from build123d import *

# Parameters (mm, degrees)
F0_R      = 20
F1_DEPTH  = 5
F2_R      = 16.6
F3_DEPTH  = 5
F4_W      = 6
F4_H      = 11
F5_DEPTH  = 2.5
F6_R      = 2
F7_SIZE   = 3
F8_W      = 2.95381
F8_H      = 3.5
F9_DEPTH  = 2.5
F10_R     = 1.25
F12_DEPTH = 0.75
F13_R     = 0.545211
F15_R     = 17.3
F15_R_2   = 16.6
F16_DEPTH = 5


with BuildPart() as f1:
    # F0 (on Top) → F1 (new body)
    with BuildSketch(Plane.XY):
        Circle(F0_R)
    extrude(amount=F1_DEPTH)

    # F2 (on face) → F3 (join)
    with BuildSketch(Plane.XY.offset(5)):
        Circle(F2_R)
    extrude(amount=F3_DEPTH)

    # F4 (on face) → F5 (join)
    with BuildSketch(Plane(origin=(0, 0, 0), x_dir=(1, 0, 0), z_dir=(0, 0, -1))):
        with Locations((0, -7.136372)):
            Rectangle(F4_W, F4_H)
    extrude(amount=F5_DEPTH)

    # F6
    f6_edges = [f1.edges().sort_by_distance(p)[0] for p in [
        (-3, 12.636372, -1.25),
        (3, 12.636372, -1.25),
        (3, 1.636372, -1.25),
        (-3, 1.636372, -1.25),
    ]]
    fillet(f6_edges, radius=F6_R)

    # F7
    f7_edges = [f1.edges().sort_by_distance(p)[0] for p in [
        (-20, 0, 0),
    ]]
    chamfer(f7_edges, length=F7_SIZE)

    # F8 (on face) → F9 (cut)
    with BuildSketch(Plane(origin=(0, 0, -2.5), x_dir=(1, 0, 0), z_dir=(0, 0, -1))):
        with Locations((0, -4.806658)):
            Rectangle(F8_W, F8_H)
        with Locations((0, -9.536388)):
            Rectangle(F8_W, F8_H)
    extrude(amount=-F9_DEPTH, mode=Mode.SUBTRACT)

    # F10
    f10_edges = [f1.edges().sort_by_distance(p)[0] for p in [
        (1.476905, 3.056658, -1.25),
        (-1.476905, 3.056658, -1.25),
        (1.476905, 6.556658, -1.25),
        (-1.476905, 6.556658, -1.25),
        (1.476905, 7.786388, -1.25),
        (-1.476905, 7.786388, -1.25),
        (-1.476905, 11.286388, -1.25),
        (1.476905, 11.286388, -1.25),
    ]]
    fillet(f10_edges, radius=F10_R)

    # F11 (on face) → F12 (cut)
    with BuildSketch(Plane(origin=(0, 0, 0), x_dir=(1, 0, 0), z_dir=(0, 0, -1))):
        with BuildLine():
            Line((5.592829, -4.637425), (6.928778, -4.637425))
            ThreePointArc((6.928778, -4.637425), (0.168305, 9.952743), (-6.79139, -4.543452))
            Line((-6.79139, -4.543452), (-5.167165, -4.543452))
            ThreePointArc((-5.167165, -4.543452), (0.331289, 8.972893), (5.592829, -4.637425))
        make_face()
    extrude(amount=-F12_DEPTH, mode=Mode.SUBTRACT)

    # F13 (on Right) → F14 (revolve)
    with BuildSketch(Plane.YZ):
        with Locations((-16.998546, 0)):
            Circle(F13_R)
    revolve(axis=Axis((0, 0, -2.59406), (0, 0, -1)))

    # F15 (on face) → F16 (join)
    with BuildSketch(Plane.XY.offset(10)):
        Circle(F15_R)
        Circle(F15_R_2, mode=Mode.SUBTRACT)
    extrude(amount=-F16_DEPTH)


solid = f1.part
Can you work these out from the model? Positions are in its coordinate system, mm. Give positions to 0.01 mm unless a question says otherwise; leave off trailing zeros. Write each loop counter-clockwise with the first axis right and the second up, starting at its lowest first coordinate (ties: lowest second). Pieces come first, ordered by that corner, then holes. Notation, with made-up numbers: M -23,58 L 6,58 A24 ccw 6,79 Z; hole C -35,-8 d1. An arc over 180 degrees is marked long. Answer in a Markdown table with one row per item. Add a question column.
Item 1: Imagine slicing it at D-D, the plane z = 6.5. Write out the boundary of the cut face in (x, y).
Item 2: For pin 1 Ø10 at (x, y) = (-8.5, -3.5) entering from -Z; pin 2 Ø0.5 at (x, z) = (0, -1) entering from -Y; pin 3 Ø0.8 at (x, z) = (6.5, 0.5) entering from -Y (3 decimals), each with a flat end and sliding along its axis, tell me the tip position at first contact or that it passes through.
Item 3: Please list where these lines run through material, in increasing order: L1, parallel to Z at x = -9, y = 9; L2, parallel to Y at x = 7, z = -0.25; L3, parallel to Y at x = 6, z = 1.5.
Item 4: Imagine slicing it at B-B, the plane y = 0. Write out the boundary of the cut face in (x, z), plus the area to 3 significant figures.
Item 5: We'd pull the mould along Y, two halves only. Please class faces 1 (the flat face through (0, 7, -2.5)), 2 (the cylindrical face through (1.12, 8.16, -1.23)): released by +Y, released by -Y, zero draft, split by the parting line, or undercut.
Item 6: Imagine slicing it at C-C, the plane z = 1.25. Write out the boundary of the cut face in (x, y), plus the area to 3 significant figures.
Item 7: Imagine slicing it at A-A, the plane z = -1.25. Write out the boundary of the cut face in (x, y).
Evaluation:
| question | item | result |
|---|---|---|
| 1 | outline | C 0,0 d34.6 |
| 2 | pin 1 | stops at z = 0 |
| 2 | pin 2 | stops at y = 1.64 |
| 2 | pin 3 | stops at y = -16.705 |
| 3 | L1 | z = 0 to 10 |
| 3 | L2 | y = -16.02 to -14.96, 14.96 to 16.02 |
| 3 | L3 | y = -17.5 to 17.5 |
| 4 | outline | M -20,3 L -17.38,0.38 A0.55 ccw long -16.45,0 L -8.72,0 L -8.72,0.75 L -7.51,0.75 L -7.51,0 L 8.03,0 L 8.03,0.75 L 8.93,0.75 L 8.93,0 L 16.45,0 A0.55 ccw long 17.38,0.38 L 20,3 L 20,5 L 17.3,5 L 17.3,10 L -17.3,10 L -17.3,5 L -20,5 Z |
| 4 | area | 364 mm² |
| 5 | face 1 | zero draft |
| 5 | face 2 | undercut |
| 6 | outline | C 0,0 d36.5 |
| 6 | area | 1,050 mm² |
| 7 | outline | M -3,3.64 A2 ccw -1,1.64 L 1,1.64 A2 ccw 3,3.64 L 3,10.64 A2 ccw 1,12.64 L -1,12.64 A2 ccw -3,10.64 Z; hole M -1.48,4.31 A1.25 ccw -0.23,3.06 L 0.23,3.06 A1.25 ccw 1.48,4.31 L 1.48,5.31 A1.25 ccw 0.23,6.56 L -0.23,6.56 A1.25 ccw -1.48,5.31 Z; hole M -1.48,9.04 A1.25 ccw -0.23,7.79 L 0.23,7.79 A1.25 ccw 1.48,9.04 L 1.48,10.04 A1.25 ccw 0.23,11.29 L -0.23,11.29 A1.25 ccw -1.48,10.04 Z |
